Input: part model. Units: mm. Frame: model coordinates. A direction names the side the tool comes from. Give positions to 0.01 mm unless a question says otherwise; leave off trailing zeros. Loops run counter-clockwise (first coordinate to the right, second up) from the corner with the lowest first, then second, coordinate; pieces in that order, holes last. Notation, with made-up numbers: (46, 0.5) -> (52, 0.5) arc R24 ccw to (52, 16.5) -> close; hole circle Ø2 at (17.5, 45.5). An arc over 180 degrees is marked (long way). Answer as a JSON object with one key per item and string values. Group by question number.
```python
from build123d import *

# Parameters (mm, degrees)
SKETCH1_W           = 70
SKETCH1_H           = 15
BOSS_EXTRUDE1_DEPTH = 2
BOSS_EXTRUDE2_START = -2
SKETCH2_R           = 7.5
BOSS_EXTRUDE2_DEPTH = 2
SKETCH3_R           = 1.8
BOSS_EXTRUDE3_DEPTH = 20
SKETCH6_R           = 0.9
CUT_EXTRUDE1_DEPTH  = 6.5


with BuildPart() as part:
    # Sketch1 → Boss-Extrude1 (new body)
    with BuildSketch(Plane(origin=(0, 0, 0), x_dir=(1, 0, 0), z_dir=(0, 1, 0))):
        with Locations((35, 7.5)):
            Rectangle(SKETCH1_W, SKETCH1_H)
    extrude(amount=BOSS_EXTRUDE1_DEPTH)

    # Sketch2 → Boss-Extrude2 (add)
    with BuildSketch(Plane(origin=(0, 2, 0), x_dir=(1, 0, 0), z_dir=(0, 1, 0)).offset(BOSS_EXTRUDE2_START)):
        with Locations((0, 7.5)):
            Circle(SKETCH2_R)
    extrude(amount=BOSS_EXTRUDE2_DEPTH)

    # Sketch3 → Boss-Extrude3 (add)
    with BuildSketch(Plane(origin=(0, 2, 0), x_dir=(1, 0, 0), z_dir=(0, 1, 0))):
        with Locations((0, 7.5)):
            Circle(SKETCH3_R)
    extrude(amount=BOSS_EXTRUDE3_DEPTH)

    # Sketch6 → Cut-Extrude1 (cut)
    with BuildSketch(Plane(origin=(0, 22, 0), x_dir=(1, 0, 0), z_dir=(0, 1, 0))):
        with Locations((0, 7.5)):
            Circle(SKETCH6_R)
    extrude(amount=-CUT_EXTRUDE1_DEPTH, mode=Mode.SUBTRACT)


solid = part.part
```
Q1. Section B-B on y = 19.5. Return the cut outline in (x, z), then the cut area to 3 significant figures.
Q2. Section C-C on x = 31. Return the cut outline in (y, z), then the cut area to 3 significant figures.
Q3. Pin query (flat end, axial travel): pin 1 Ø3 at (y, z) = (16.5, -10.5) entering from -X (3 decimals); pin 2 Ø8 at (x, z) = (29, -3) entering from +Y; pin 3 Ø6 at (y, z) = (19, -3) entering from +X (3 decimals). Return the tip coordinate at first contact, or that it passes through.
Q4. Section D-D on y = 9. Return the cut outline in (x, z), then the cut area to 3 significant figures.
Q5. Set-up query: faces 4 (the face through (70, 1, -7)), 5 (the face through (-0.12, 18.8, -8.39)). Return all of +Z, -Z, +X, -X, +Y, -Y with unobstructed straight access to the full face (end or side cutting, diameter ignored); none if empty.
Q6. Ray query, probe 1 along Z at (x, y) = (0, 19.5); probe 2 along X at (y, z) = (17.75, -7.5); probe 3 along Y at (x, z) = (0, -5.5). Return the intervals inside material, ascending.
Q7. Section A-A on z = -7.5. Return the cut outline in (x, y), then the cut area to 3 significant figures.
Q8. Pull-direction query (X, two-part tool) for faces 1 (the face through (0, 15.5, -8)), 2 (the face through (-7.5, 0.99, -7.66)), 3 (the face through (-1, 22, -7)); classes: +X half, -X half, draft (parallel to the pull), parting line (faces both ways), or undercut.
Numbers:
{
 "1": {"outline": "circle Ø3.6 at (0, -7.5); hole circle Ø1.8 at (0, -7.5)", "area": "7.63 mm²"},
 "2": {"outline": "(0, -15) -> (2, -15) -> (2, 0) -> (0, 0) -> close", "area": "30.0 mm²"},
 "3": {"pin 1": "stops at x = -0.995", "pin 2": "stops at y = 2", "pin 3": "stops at x = 0.995"},
 "4": {"outline": "circle Ø3.6 at (0, -7.5)", "area": "10.2 mm²"},
 "5": {"face 4": "+Z, -Z, +X, +Y, -Y", "face 5": "+Y"},
 "6": {"probe 1": "z = -9.3 to -8.4, -6.6 to -5.7", "probe 2": "x = -1.8 to -0.9, 0.9 to 1.8", "probe 3": "y = 0 to 2"},
 "7": {"outline": "(-7.5, 0) -> (70, 0) -> (70, 2) -> (1.8, 2) -> (1.8, 22) -> (0.9, 22) -> (0.9, 15.5) -> (-0.9, 15.5) -> (-0.9, 22) -> (-1.8, 22) -> (-1.8, 2) -> (-7.5, 2) -> close", "area": "215 mm²"},
 "8": {"face 1": "undercut", "face 2": "-X half", "face 3": "draft"}
}
